```python
from build123d import *

# Parameters (mm, degrees)
BOSS_EXTRUDE1_DEPTH      = 50
SKETCH3_W                = 5
SKETCH3_H                = 50
BOSS_EXTRUDE3_DEPTH      = 180
CORTE_EXTRUS_O1_DEPTH    = 10
ESBO_O3_W                = 50
ESBO_O3_H                = 7.5
RESSALTO_EXTRUS_O2_DEPTH = 10
ESBO_O4_W                = 7.5
ESBO_O4_H                = 45
CORTE_EXTRUS_O2_DEPTH    = 10
CORTE_EXTRUS_O3_START    = -20
CORTE_EXTRUS_O3_DEPTH    = 170
ESBO_O6_R                = 0.6
CORTE_EXTRUS_O4_DEPTH    = 195
PADR_O_LINEAR1_COUNT     = 2
PADR_O_LINEAR1_PITCH     = 39


with BuildPart() as part:
    # Sketch1 → Boss-Extrude1 (new body)
    with BuildSketch(Plane.XY):
        Polygon((0, 0), (0, 30), (12.8, 30), (12.8, 0), (7.8, 0), (7.8, 10), (6, 10), (6, 0), align=None)
    extrude(amount=BOSS_EXTRUDE1_DEPTH)

    # Sketch3 → Boss-Extrude3 (add)
    with BuildSketch(Plane.XZ):
        with Locations((10.3, 25)):
            Rectangle(SKETCH3_W, SKETCH3_H)
    extrude(amount=BOSS_EXTRUDE3_DEPTH)

    # Esboço2 → Corte-extrusão1 (cut)
    with BuildSketch(Plane.XZ):
        with BuildLine():
            Line((6, 50), (6, 0))
            ThreePointArc((6, 0), (2.708949196, 25), (6, 50))
        make_face()
    extrude(amount=-CORTE_EXTRUS_O1_DEPTH, mode=Mode.SUBTRACT)

    # Esboço3 → Ressalto-extrusão2 (add)
    with BuildSketch(Plane.ZY):
        with Locations((25, 26.25)):
            Rectangle(ESBO_O3_W, ESBO_O3_H)
    extrude(amount=RESSALTO_EXTRUS_O2_DEPTH)

    # Esboço4 → Corte-extrusão2 (cut)
    with BuildSketch(Plane.XZ.offset(-22.5)):
        with Locations((-3.75, 25)):
            Rectangle(ESBO_O4_W, ESBO_O4_H)
    extrude(amount=-CORTE_EXTRUS_O2_DEPTH, mode=Mode.SUBTRACT)

    # Esboço5 → Corte-extrusão3 (cut)
    with BuildSketch(Plane(origin=(0, 30, 0), x_dir=(1, 0, 0), z_dir=(0, 1, 0)).offset(CORTE_EXTRUS_O3_START)):
        with BuildLine():
            Line((12.8, -41.5000945), (12.8, -47.5))
            ThreePointArc((12.8, -47.5), (9.816837413, -44.50004725), (12.8, -41.5000945))
        make_face()
    corte_extrus_o3 = extrude(amount=-CORTE_EXTRUS_O3_DEPTH, mode=Mode.SUBTRACT)

    # Esboço6 → Corte-extrusão4 (cut)
    with BuildSketch(Plane(origin=(0, 30, 0), x_dir=(1, 0, 0), z_dir=(0, 1, 0))):
        with Locations(Location((11.3, -44.5, 0), (0, 0, 270))):
            Circle(ESBO_O6_R)
    corte_extrus_o4 = extrude(amount=-CORTE_EXTRUS_O4_DEPTH, mode=Mode.SUBTRACT)

    # Padrão linear1: Corte-extrusão3, Corte-extrusão4 ×2
    with Locations(*[(0, 0, -i * PADR_O_LINEAR1_PITCH) for i in range(1, PADR_O_LINEAR1_COUNT)]):
        add(corte_extrus_o3, mode=Mode.SUBTRACT)
        add(corte_extrus_o4, mode=Mode.SUBTRACT)


solid = part.part
```
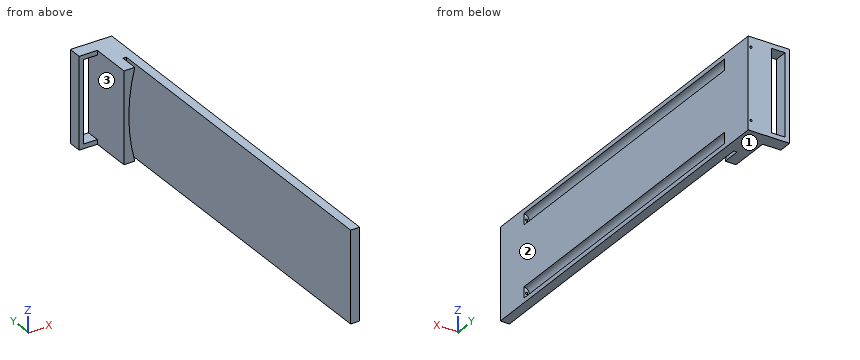
Input: part model. Units: mm. Frame: model coordinates. Face numbers are marked on the shaded views. Give positions to 0.01 mm unless a question says otherwise; leave off trailing zeros. Loops run counter-clockwise (first coordinate to the right, second up) from the corner with the lowest first, then second, coordinate; pieces in that order, holes last.
1) Section query B-B on z = 30. Return the cut outline in (x, y).
A:
outline: (-10, 22.5) - (-7.5, 22.5) - (-7.5, 30) - (-10, 30) - close; (0, 0) - (2.84, 0) - (2.84, 10) - (7.8, 10) - (7.8, -180) - (12.8, -180) - (12.8, 30) - (0, 30) - close
2) Contact query for flat-ended pins moving along their axis: pin 1 (1 mm diameter, centred on x = 11.3, z = 5.5, fed in from +Y); pin 2 (3 mm diameter, centred on x = 3, z = 22.5, fed in from -Y); pin 3 (2 mm diameter, centred on y = 0, z = 17, fed in from -X). Output: stop coordinate, or through.
A:
pin 1: stops at y = -165
pin 2: stops at y = 0
pin 3: stops at x = 0
3) Mould query, pull axis X, two halves, no side actions, for the marked faces 1, 2 and 3. Classes: released by +X, released by -X, zero draft, split by the parting line, or undercut.
A:
face 1: zero draft
face 2: released by +X
face 3: undercut
4) Section query A-A on x = -4.25. Return the cut outline in (y, z), and give its area (3 significant figures).
A:
outline: (22.5, 0) - (30, 0) - (30, 2.5) - (22.5, 2.5) - close; (22.5, 47.5) - (30, 47.5) - (30, 50) - (22.5, 50) - close
area: 37.5 mm2
5) Section query D-D on z = 21.5. Return the cut outline in (x, y), and give its area (3 significant figures).
A:
outline: (-10, 22.5) - (-7.5, 22.5) - (-7.5, 30) - (-10, 30) - close; (0, 0) - (2.77, 0) - (2.77, 10) - (7.8, 10) - (7.8, -180) - (12.8, -180) - (12.8, 30) - (0, 30) - close
area: 1,250 mm2
6) Line query: L1, parallel to X at y = 23, z = 44; L2, parallel to X at y = 16.75, z = 5.5; L3, parallel to X at y = -50.5, z = 21.5. Output: solid intervals per line, ascending.
A:
L1: x = -10 to -7.5, 0 to 10.97, 11.63 to 12.8
L2: x = 0 to 10.7, 11.9 to 12.8
L3: x = 7.8 to 12.8
7) Section query C-C on y = -75.5. Return the cut outline in (x, z), and give its area (3 significant figures).
A:
outline: (7.8, 0) - (12.8, 0) - (12.8, 2.5) arc R3 cw to (12.8, 8.5) - (12.8, 41.5) arc R3 cw to (12.8, 47.5) - (12.8, 50) - (7.8, 50) - close
area: 222 mm2
